Autodesk Inventor part; units mm, degrees
ref_plane "YZ Plane" through (0, 0, 0) normal (1, 0, 0) x (0, 1, 0)
ref_plane "XZ Plane" through (0, 0, 0) normal (0, 1, 0) x (-1, 0, 0)
ref_plane "XY Plane" through (0, 0, 0) normal (0, 0, 1) x (1, 0, 0)
sketch "Sketch1" plane through (0, 0, 0) normal (0, 0, 1) x (1, 0, 0)
  circle A0 centre (0, 0) radius 70
  circle A1 centre (0, 0) radius 8.5
  circle A2 centre (0, 0) radius 40
  dimension "d0" = 140
  dimension "d1" = 17
  dimension "d2" = 80
extrude "Extrusion1" add sketch "Sketch1" against normal blind 7 contours A0 | A1 | A2
extrude "Extrusion2" add sketch "Sketch1" along normal blind 40 contours A2
properties part number "47T-Sprocket"
Input: part model. Units: mm. Frame: model coordinates. A direction names the side the tool comes from. Coordinates: 2 decimals unless noted, no trailing zeros. Loops run counter-clockwise (first coordinate to the right, second up) from the corner with the lowest first, then second, coordinate; pieces in that order, holes last. Notation, with made-up numbers: (75, 43.25) - (122, 43.25) arc R14 ccw to (122, 58.25) - close; hole circle Ø8 at (-14.75, -7.5). An arc over 180 degrees is marked (long way). Answer in a Markdown table with one row per item.
(1) Mould query, pull axis Y, two halves, no side actions, for faces 1 (the face through (-55.55, -42.594, -3.451)), 2 (the face through (-1, 9, 40)), 3 (the face through (4.57, -7.167, 19.72)). Classes: pulls with the +Y half, pulls with the -Y half, needs draft (parallel to the pull), parting line crosses it, or undercut.
Model answer:
| item | result |
|---|---|
| face 1 | parting line crosses it |
| face 2 | needs draft |
| face 3 | undercut |
(2) Pin query (flat end, axial travel): P1, Ø6, axis at y = 27, z = 19.5, coming from the +X side; P2, Ø1, axis at x = -30.5, z = 17, coming from the +Y side; P3, Ø3, axis at y = -33, z = -2, coming from the +X side. Return the tip coordinate at first contact, or that it passes through.
Model answer:
| item | result |
|---|---|
| P1 | stops at x = 32 |
| P2 | stops at y = 26.46 |
| P3 | stops at x = 62.51 |
(3) Material intervals for L1, parallel to Y at x = 0, z = 17.5; L2, parallel to Z at x = 0, y = 6; L3, parallel to Y at x = 4, z = 7.5, sorted ascending. Write a range as from..to.
Model answer:
| item | result |
|---|---|
| L1 | y = -40..-8.5, 8.5..40 |
| L2 | z = -7..0 |
| L3 | y = -39.8..-7.5, 7.5..39.8 |
(4) Cut plane A-A on y = 0. Output: boundary loops of the cut face in (x, z), plus the area to 3 significant figures.
Model answer:
| item | result |
|---|---|
| outline | (-70, -7) - (70, -7) - (70, 0) - (40, 0) - (40, 40) - (8.5, 40) - (8.5, 0) - (-8.5, 0) - (-8.5, 40) - (-40, 40) - (-40, 0) - (-70, 0) - close |
| area | 3,500 mm² |
(5) Cut plane C-C on z = 11.5. Output: boundary loops of the cut face in (x, y).
Model answer:
| item | result |
|---|---|
| outline | circle Ø80 at (0, 0); hole circle Ø17 at (0, 0) |
(6) Cut plane D-D on y = -22.5. Output: boundary loops of the cut face in (x, z), plus the area to 3 significant figures.
Model answer:
| item | result |
|---|---|
| outline | (-66.29, -7) - (66.29, -7) - (66.29, 0) - (33.07, 0) - (33.07, 40) - (-33.07, 40) - (-33.07, 0) - (-66.29, 0) - close |
| area | 3,570 mm² |
(7) Set-up query: faces 4 (the face through (-1, 1, -7)), 5 (the face through (30, -30, 0)). Return all of +Z, -Z, +X, -X, +Y, -Y with unobstructed straight access to the full face (end or side cutting, diameter ignored); none if empty.
Model answer:
| item | result |
|---|---|
| face 4 | -Z, +X, -X, +Y, -Y |
| face 5 | +Z |
